Here's how the part is built. I have some questions about the finished solid (model axes, mm). Face numbers are marked on the shaded views. A direction names the side the tool comes from. Coordinates: 2 decimals unless noted, no trailing zeros. Order: outer loops, then holes, each group sorted by start corner. A loop starts at its lowest first (then second) coordinate and runs counter-clockwise, first axis right, second up. Notation, with made-up numbers: (12, 25.5) - (39, 25.5) arc R33 ccw to (39, 60.5) - close; hole circle Ø9 at (42, 63). An arc over 180 degrees is marked (long way). Answer in a Markdown table with one row per item. Add a question column.
Item 1: Will these pins go through, and if not, where does the flat tip stop? pin 1 Ø0.8 at (x, y) = (-0.5, -0.5) entering from -Z; pin 2 Ø4 at (x, y) = (3.5, 3) entering from -Z; pin 3 Ø1 at (y, z) = (-1.5, 7.5) entering from +X.
Item 2: If I drill on line 1 along Y through (x, z) = (0, 4) (3 decimals); line 2 along X through (y, z) = (-1, 8.75); line 3 along X through (y, z) = (-0.5, 3.75), over which ranges is the centre line in solid material (lowest first)? Write a range as from..to.
Item 3: I want a section at A-A (x = 0). Please give me the cut outline in (y, z) (3 decimals), plus the area to 3 significant figures.
Item 4: I want a section at D-D (y = -2.75). Please give me the cut outline in (x, z).
Item 5: Thinking about a two-plate mould opening in X: for the marked faces 3, 4 and 5, which applies, +X half, -X half, draft (parallel to the pull), parting line (faces both ways), or undercut?
Item 6: On a 3-axis mill with a long thin cutter (end or side, diameter ignored), from which of +Z, -Z, +X, -X, +Y, -Y can I reach the whole of each face in a straight line? I mean the marked faces 1 and 2. Say none if no direction works.
Item 7: I want a section at C-C (y = 0.75). Please give me the cut outline in (x, z), plus the area to 3 significant figures.
Item 8: I want a section at B-B (z = 3.5). Please give me the cut outline in (x, y) (3 decimals), plus the area to 3 significant figures.
```python
from build123d import *

# Parameters (mm, degrees)
BOSS_EXTRUDE1_DEPTH = 10
CUT_EXTRUDE1_DEPTH  = 9


with BuildPart() as part:
    # Sketch1 → Boss-Extrude1 (new body)
    with BuildSketch(Plane.XY):
        Polygon((4.618802154, 0), (2.309401077, 4), (-2.309401077, 4), (-4.618802154, 0), (-2.309401077, -4), (2.309401077, -4), align=None)
    extrude(amount=BOSS_EXTRUDE1_DEPTH)

    # Sketch2 → Cut-Extrude1 (cut)
    with BuildSketch(Plane(origin=(0, 0, 0), x_dir=(-1, 0, 0), z_dir=(0, 0, -1))):
        with BuildLine():
            Line((-1.11, 1.045717457), (1.11, 1.045717457))
            ThreePointArc((1.11, 1.045717457), (0, -1.525), (-1.11, 1.045717457))
        make_face()
    extrude(amount=-CUT_EXTRUDE1_DEPTH, mode=Mode.SUBTRACT)


solid = part.part
```
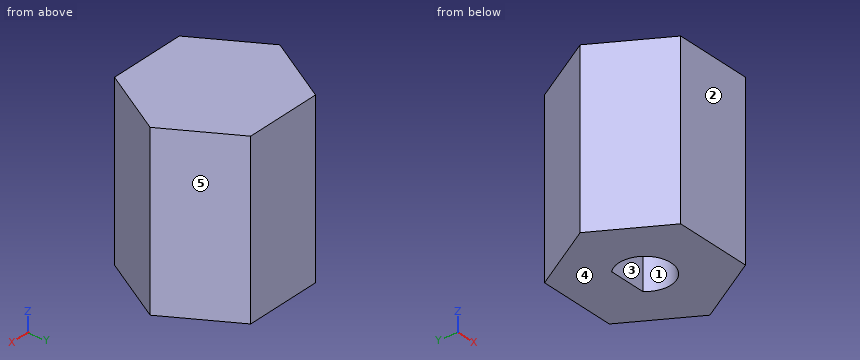
Values follow:
| question | item | result |
|---|---|---|
| 1 | pin 1 | stops at z = 9 |
| 1 | pin 2 | stops at z = 0 |
| 1 | pin 3 | stops at x = 4.04 |
| 2 | line 1 | y = -4..-1.525, 1.046..4 |
| 2 | line 2 | x = -4.04..-1.15, 1.15..4.04 |
| 2 | line 3 | x = -4.33..-1.44, 1.44..4.33 |
| 3 | outline | (-4, 0) - (-1.525, 0) - (-1.525, 9) - (1.046, 9) - (1.046, 0) - (4, 0) - (4, 10) - (-4, 10) - close |
| 3 | area | 56.9 mm^2 |
| 4 | outline | (-3.03, 0) - (3.03, 0) - (3.03, 10) - (-3.03, 10) - close |
| 5 | face 3 | undercut |
| 5 | face 4 | draft |
| 5 | face 5 | +X half |
| 6 | face 1 | -Z |
| 6 | face 2 | +Z, -Z, +X, -X, -Y |
| 7 | outline | (-4.19, 0) - (-1.33, 0) - (-1.33, 9) - (1.33, 9) - (1.33, 0) - (4.19, 0) - (4.19, 10) - (-4.19, 10) - close |
| 7 | area | 59.8 mm^2 |
| 8 | outline | (-4.619, 0) - (-2.309, -4) - (2.309, -4) - (4.619, 0) - (2.309, 4) - (-2.309, 4) - close; hole (-1.11, 1.046) arc R1.525 ccw (long way) to (1.11, 1.046) - close |
| 8 | area | 48.9 mm^2 |
